For this review, use the dimensioned drawing (mm, ordinates from the lowest corner) and the shaded views. A direction names the side the tool comes from. Give positions to 0.01 mm unless a question says otherwise; leave off trailing zeros. Loops run counter-clockwise (first coordinate to the right, second up) from the corner with the lowest first, then second, coordinate; pieces in that order, holes last. Notation, with made-up numbers: (25, 87) -> (30, 87) arc R27 cw to (30, 103) -> close; hole circle Ø9 at (64, -11). An arc over 180 degrees is marked (long way). Write each question's results on one line, items separated by ' | '. Start each with the question number.
Q1. We need section B-B (x = 43). Write out the cut boundary in (y, z), plus the area to 3 significant figures.
Q2. Mouldability with a two-part tool opening along Y and no side actions: class the marked faces 4, 5 and 6 as released by +Y, released by -Y, zero draft, split by the parting line, or undercut.
Q3. We need section C-C (y = 45). Write out the cut boundary in (x, z) (1 decimal), plus the area to 3 significant figures.
Q4. We need section D-D (y = 28). Write out the cut boundary in (x, z) (1 decimal), plus the area to 3 significant figures.
Q5. Wall thickness on L1, parallel to X at y = 85, z = 19.5 (1 decimal); L2, parallel to X at y = 42, z = 24.5 (1 decimal); L3, parallel to Y at x = 37, z = 19 (1 decimal): over which ranges is each line inside the solid? List them lowest first. Write a range as [from, to].
Q6. Machinability: for the marked faces 1, 2 and 3, which of the approach directions +Z, -Z, +X, -X, +Y, -Y give a long, thin tool a straight path to every point of the face, cutting with its end or side? Answer none if there is none.
Q7. Insertion check: pin 1 Ø3 at (y, z) = (46, 65.5) entering from +X; pin 2 Ø3.5 at (x, y) = (34.5, 7) entering from -Z; pin 3 Ø3.5 at (x, y) = (34, 7.5) entering from +Z. Each pin has a flat end and moves straight along its axis. Give the tip position at first contact, or say it passes through.
Q8. We need section A-A (z = 39). Write out the cut boundary in (x, y) (1 decimal), plus the area to 3 significant figures.
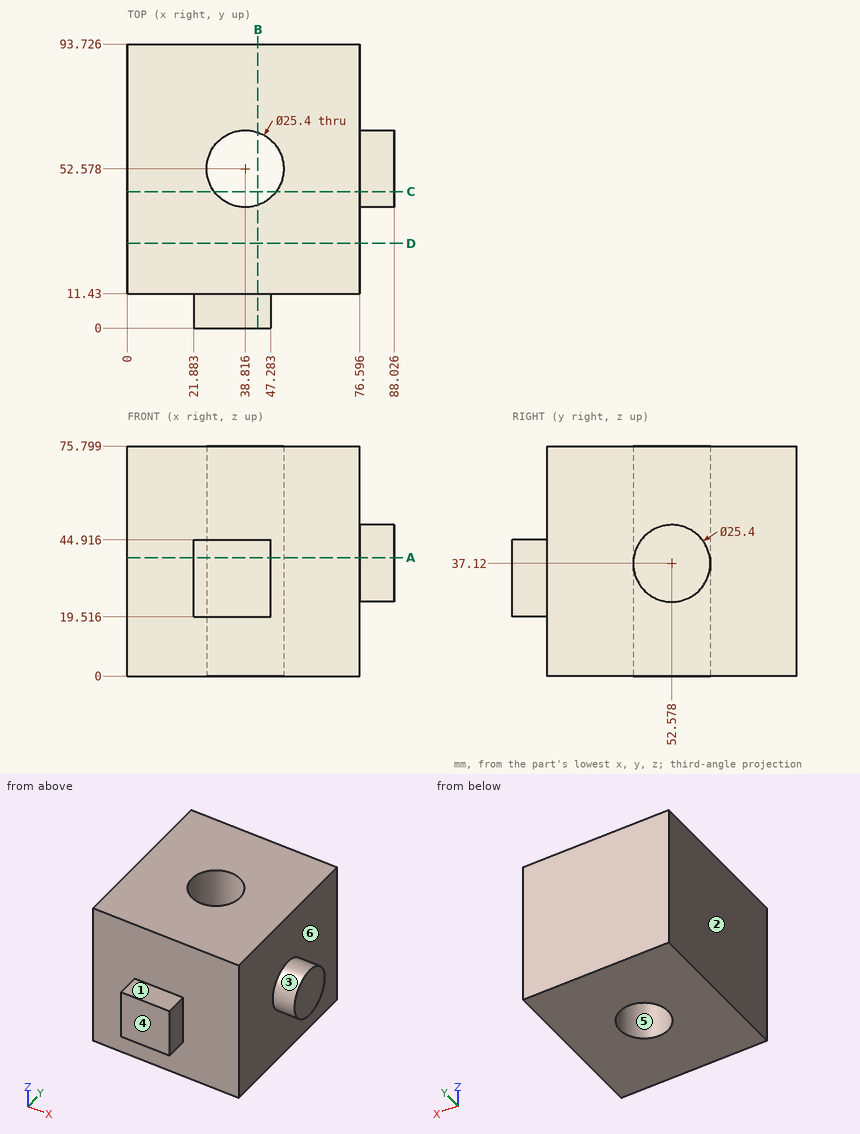
Output:
1) outline: (0, 19.52) -> (11.43, 19.52) -> (11.43, 0) -> (40.59, 0) -> (40.59, 75.8) -> (11.43, 75.8) -> (11.43, 44.92) -> (0, 44.92) -> close; (64.57, 0) -> (93.73, 0) -> (93.73, 75.8) -> (64.57, 75.8) -> close | area: 4,710 mm2
2) face 4: released by -Y | face 5: undercut | face 6: zero draft
3) outline: (0, 0) -> (28.6, 0) -> (28.6, 75.8) -> (0, 75.8) -> close; (49, 0) -> (76.6, 0) -> (76.6, 26.9) -> (88, 26.9) -> (88, 47.3) -> (76.6, 47.3) -> (76.6, 75.8) -> (49, 75.8) -> close | area: 4,490 mm2
4) outline: (0, 0) -> (76.6, 0) -> (76.6, 75.8) -> (0, 75.8) -> close | area: 5,810 mm2
5) L1: [0, 76.6] | L2: [0, 31.8], [45.8, 76.6] | L3: [11.4, 40], [65.1, 93.7]
6) face 1: +Z, +X, -X, -Y | face 2: +Z, -Z, -X, +Y, -Y | face 3: +X
7) pin 1: x = 76.6 | pin 2: z = 19.52 | pin 3: z = 44.92
8) outline: (0, 11.4) -> (21.9, 11.4) -> (21.9, 0) -> (47.3, 0) -> (47.3, 11.4) -> (76.6, 11.4) -> (76.6, 40) -> (88, 40) -> (88, 65.1) -> (76.6, 65.1) -> (76.6, 93.7) -> (0, 93.7) -> close; hole circle Ø25.4 at (38.8, 52.6) | area: 6,370 mm2
